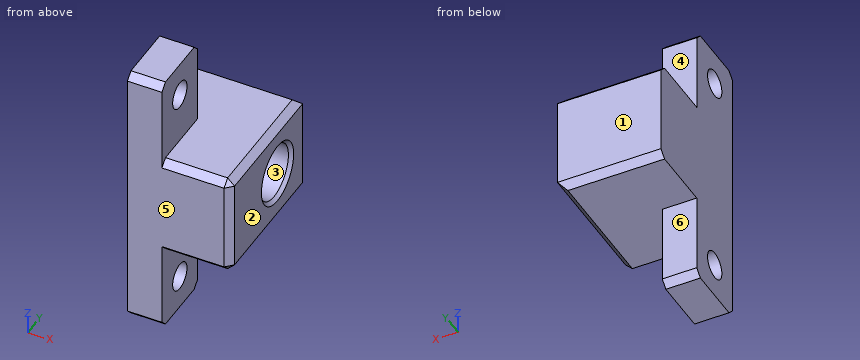
Autodesk Inventor part; units mm, degrees
ref_plane "YZ Plane" through (0, 0, 0) normal (1, 0, 0) x (0, 1, 0)
ref_plane "XZ Plane" through (0, 0, 0) normal (0, 1, 0) x (-1, 0, 0)
ref_plane "XY Plane" through (0, 0, 0) normal (0, 0, 1) x (1, 0, 0)
sketch "Sketch1" plane through (0, 0, 0) normal (1, 0, 0) x (0, 1, 0)
  line L0 (-5, 20) -> (5, 20)
  line L1 (5, 20) -> (5, -20)
  line L2 (5, -20) -> (-5, -20)
  line L3 (-5, -20) -> (-5, 20)
  line L4 (-5, 20) -> (5, -20) construction
  line L5 (5, 20) -> (-5, -20) construction
  line L6 (-7.5, 7.5) -> (7.5, -7.5) construction
  line L7 (7.5, 7.5) -> (-7.5, -7.5) construction
  line L8 (15, -7.5) -> (15, 7.5)
  line L9 (15, 7.5) -> (-5, 7.5)
  line L10 (-15, -7.5) -> (15, 7.5) construction
  line L11 (15, -7.5) -> (-15, 7.5) construction
  line L12 (-5, -7.5) -> (15, -7.5)
  point P0 (0, 0)
  point P1 (5, -7.5)
  point P2 (5, 7.5)
  point P3 (5, -7.5)
  dimension "d0" = 10
  dimension "d1" = 40
  dimension "d3" = 15
  dimension "d32" = 10
  dimension "d33" = 40
extrude "Extrusion1" add sketch "Sketch1" along normal blind 5
sketch "Sketch4" plane through (0, 0, 0) normal (-1, 0, 0) x (0, 0, 1)
  line L0 (-20, -5) -> (-20, 5)
  line L1 (-20, 0) -> (-17, 0)
  line L2 (-17, 0) -> (-15, 0)
  circle A0 centre (-15, 0) radius 2
  line L3 (20, 5) -> (20, -5)
  circle A1 centre (15, 0) radius 2
  point P0 (0, 0)
  point P1 (-20, -4)
  point P2 (-20, 4)
  point P3 (20, 4)
  point P4 (20, -4)
  dimension "d25" = 3
  dimension "d26" = 2
  dimension "d28" = 4
extrude "Extrusion4" cut sketch "Sketch4" against normal blind 10
sketch "Sketch5" plane through (5, 0, 0) normal (1, 0, 0) x (0, 0, -1)
  line L0 (7.5, 15) -> (-7.5, 15)
  line L1 (-7.5, 15) -> (-7.5, -5)
  line L2 (-20, -5) -> (20, -5)
  line L3 (-7.5, 15) -> (7.5, 15)
  line L4 (7.5, 5) -> (7.5, 15)
  line L5 (7.5, 5) -> (7.5, 15)
  line L6 (7.5, 15) -> (7.5, 5)
  line L7 (7.5, -5) -> (-7.5, -5)
  line L8 (7.5, 5) -> (7.5, -5)
  line L9 (-7.5, -5) -> (7.5, -5)
  point P0 (0, 0)
extrude "Extrusion5" add sketch "Sketch5" along normal blind 10
sketch "Sketch6" plane through (15, 0, 0) normal (1, 0, 0) x (0, 0, -1)
  line L0 (7.5, 15) -> (-7.5, 15)
  circle A0 centre (0, 8) radius 4
  point P0 (0, 0)
  point P1 (0, 15)
  dimension "d37" = 8
  dimension "d40" = 7
extrude "Extrusion6" cut sketch "Sketch6" against normal blind 10
thread "Thread2"
chamfer "Chamfer5" distance 1 angle 45 11 edges at (7.5, 15, 7.5) (7.5, 15, -7.5) (15, 5, -7.5) (15, 5, 7.5) (15, -5, 0) (10, -5, 7.5) (2.5, 5, 20) (2.5, -5, 20) (2.5, 5, -20) (2.5, -5, -20) (10, -5, -7.5)
chamfer "Chamfer6" distance 0.5 angle 45 1 edges at (15, 8, 4)
properties part number "chain piston adaptor"
Check sheet for the modelled part. Datum: model origin and axes. Units: mm. Face numbers are marked on the shaded views. A direction names the side the tool comes from. Round coordinates to 2 decimals unless told otherwise and drop trailing zeros. Order: outer loops, then holes, each group sorted by start corner. A loop starts at its lowest first (then second) coordinate and runs counter-clockwise, first axis right, second up.
Q1. Cross-section at C-C, the plane z = 0. Enter the section's corners in (x, y), plus the area to 3 significant figures.
Filled sheet:
outline: (0, -5) - (14, -5) - (15, -4) - (15, 3.5) - (14.5, 4) - (5, 4) - (5, 12) - (14.5, 12) - (15, 12.5) - (15, 15) - (0, 15) - close
area: 219 mm2
Q2. Cross-section at A-A, the plane y = 0. Enter the section's corners in (x, z), plus the area to 3 significant figures.
Filled sheet:
outline: (0, -20) - (5, -20) - (5, -17) - (0, -17) - close; (0, -13) - (5, -13) - (5, -7.5) - (14, -7.5) - (15, -6.5) - (15, 6.5) - (14, 7.5) - (5, 7.5) - (5, 13) - (0, 13) - close; (0, 17) - (5, 17) - (5, 20) - (0, 20) - close
area: 309 mm2
Q3. Cross-section at B-B, the plane x = 2.75. Enter the section's corners in (y, z), plus the area to 3 significant figures.
Filled sheet:
outline: (-5, -19) - (-4, -20) - (4, -20) - (5, -19) - (5, -7.5) - (14, -7.5) - (15, -6.5) - (15, 6.5) - (14, 7.5) - (5, 7.5) - (5, 19) - (4, 20) - (-4, 20) - (-5, 19) - close; hole circle Ø4 at (0, -15); hole circle Ø4 at (0, 15)
area: 522 mm2
Q4. Draft check along Y on the marked faces 1, 2 and 3. Enter one of: pulls with the +Y half, pulls with the -Y half, needs draft (parallel to the pull), parting line crosses it, or undercut.
Filled sheet:
face 1: pulls with the +Y half
face 2: needs draft
face 3: undercut
Q5. Cross-section at D-D, the plane x = 8.5. Enter the section's corners in (y, z).
Filled sheet:
outline: (-5, -6.5) - (-4, -7.5) - (14, -7.5) - (15, -6.5) - (15, 6.5) - (14, 7.5) - (-4, 7.5) - (-5, 6.5) - close; hole circle Ø8 at (8, 0)
Q6. Depth check by flat-ended pin: P1, Ø4, axis at x = 3, z = 13.5, coming from the +Y side; P2, Ø1, axis at x = 4, y = 13, coming from the -Z side; P3, Ø8, axis at y = 1.5, z = -11, coming from the +X side; P4, Ø1, axis at y = 4.5, z = -12, coming from the -X side. Enter the tip coordinate at first touch or a pass-through.
Filled sheet:
P1: stops at y = 5
P2: stops at z = -7.5
P3: stops at x = 14.5
P4: stops at x = 0
Q7. Set-up check for the marked faces 4, 5 and 6: record each of +Z, -Z, +X, -X, +Y, -Y from which the full face is reachable in a straight line by a thin tool's end or side.
Filled sheet:
face 4: +Z, +X, -X, +Y
face 5: +Z, -Z, +X, -X, -Y
face 6: -Z, +X, -X, +Y
Q8. Scan lines: L1, parallel to Y at x = 3.2, z = -15; L2, parallel to Y at x = 12, z = 0; L3, parallel to X at y = 3.5, z = 15.5. Record each from-to range of solid material in increasing order.
Filled sheet:
L1: y = -5 to -2, 2 to 5
L2: y = -5 to 4, 12 to 15
L3: x = 0 to 5
